Part model, mm, in its own coordinate system. Face numbers are marked on the shaded views. A direction names the side the tool comes from. Round coordinates to 2 decimals unless told otherwise and drop trailing zeros. Loops run counter-clockwise (first coordinate to the right, second up) from the corner with the lowest first, then second, coordinate; pieces in that order, holes last. Notation, with made-up numbers: (30, -32.75) -> (69, -32.75) arc R9 ccw to (69, -22.75) -> close; hole circle Ø2 at (68.25, 61.25). An arc over 180 degrees is marked (long way). Answer as a JSON object with one key per item and string values. Group by question number.
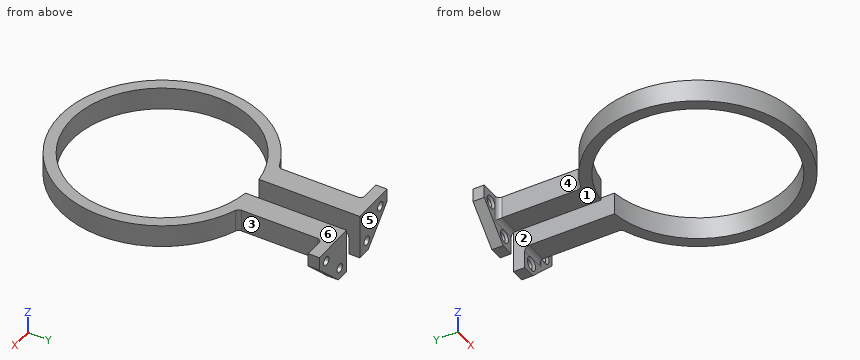
from build123d import *
from OCP.BRepFilletAPI import BRepFilletAPI_MakeChamfer

# Parameters (mm, degrees)
BOSS_EXTRUDE1_DEPTH = 12.7
SKETCH2_W           = 25.4
SKETCH2_H           = 25.4
SKETCH2_R           = 2.54
BOSS_EXTRUDE2_DEPTH = 6.35
CHAMFER2_SIZE       = 1.27
CHAMFER2_SIZE2      = 1.103994157
CHAMFER3_SIZE       = 17.78
FILLET3_R           = 2.54


with BuildPart() as part:
    # Sketch1 → Boss-Extrude1 (new body)
    with BuildSketch(Plane.XY):
        with BuildLine():
            Line((-6.35, 51.041519619), (-6.35, 101.841519619))
            Line((-6.35, 101.841519619), (-19.05, 101.841519619))
            Line((-19.05, 101.841519619), (-19.05, 54.554593986))
            ThreePointArc((-19.05, 54.554593986), (0, -57.785), (19.05, 54.554593986))
            Line((19.05, 54.554593986), (19.05, 101.841519619))
            Line((19.05, 101.841519619), (6.35, 101.841519619))
            Line((6.35, 101.841519619), (6.35, 51.041519619))
            ThreePointArc((6.35, 51.041519619), (0, -51.435), (-6.35, 51.041519619))
        make_face()
    extrude(amount=BOSS_EXTRUDE1_DEPTH)

    # Sketch2 → Boss-Extrude2 (add)
    with BuildSketch(Plane(origin=(0, 101.841519619, 0), x_dir=(1, 0, 0), z_dir=(0, 1, 0))):
        with Locations((-19.05, 0)):
            Rectangle(SKETCH2_W, SKETCH2_H)
        with Locations(Location((-25.4, -6.35, 0), (0, 0, 270))):
            Circle(SKETCH2_R, mode=Mode.SUBTRACT)
        with Locations(Location((-12.7, 6.35, 0), (0, 0, 270))):
            Circle(SKETCH2_R, mode=Mode.SUBTRACT)
    boss_extrude2 = extrude(amount=BOSS_EXTRUDE2_DEPTH)

    # Mirror5: Boss-Extrude2 across plane
    add(boss_extrude2.mirror(Plane(origin=(0, 0, 0), x_dir=(0, 0, 1), z_dir=(1, 0, 0))))

    # Chamfer2: one chamfer whose edges measure the first distance from different faces: ONE call of the kernel's chamfer builder (chamfer() names one face for all edges)
    chamfer2_edges_1 = [part.edges().sort_by_distance(p)[0] for p in [
        (-12.7, 101.841519619, -8.89),
    ]]
    chamfer2_side_1 = [part.faces().sort_by_distance(p)[0] for p in [
        (-12.7, 105.016519619, -8.89),
    ]]
    chamfer2_edges_2 = [part.edges().sort_by_distance(p)[0] for p in [
        (-25.4, 101.841519619, 3.81),
    ]]
    chamfer2_side_2 = [part.faces().sort_by_distance(p)[0] for p in [
        (-25.4, 105.016519619, 3.81),
    ]]
    chamfer2_edges_3 = [part.edges().sort_by_distance(p)[0] for p in [
        (12.7, 101.841519619, -8.89),
        (25.4, 101.841519619, 3.81),
    ]]
    chamfer2_side_3 = [part.faces().sort_by_distance(p)[0] for p in [
        (21.360206035, 101.841519619, -2.310206035),
    ]]
    chamfer2 = BRepFilletAPI_MakeChamfer(part.part.solid().wrapped)
    for e in chamfer2_edges_1:
        chamfer2.Add(CHAMFER2_SIZE, CHAMFER2_SIZE2, e.wrapped, chamfer2_side_1[0].wrapped)  # the first distance lies on this face
    for e in chamfer2_edges_2:
        chamfer2.Add(CHAMFER2_SIZE, CHAMFER2_SIZE2, e.wrapped, chamfer2_side_2[0].wrapped)  # the first distance lies on this face
    for e in chamfer2_edges_3:
        chamfer2.Add(CHAMFER2_SIZE, CHAMFER2_SIZE2, e.wrapped, chamfer2_side_3[0].wrapped)  # the first distance lies on this face
    add(Compound.cast(chamfer2.Shape()), mode=Mode.REPLACE)

    # Chamfer3
    chamfer3_edges = [part.edges().sort_by_distance(p)[0] for p in [
        (-31.75, 105.016519619, -12.7),
        (31.75, 105.016519619, -12.7),
    ]]
    chamfer(chamfer3_edges, length=CHAMFER3_SIZE)

    # Fillet3
    fillet3_edges = [part.edges().sort_by_distance(p)[0] for p in [
        (12.7, 101.841519619, 0),
        (-19.05, 54.554593986, 6.35),
        (-19.05, 101.841519619, 6.35),
        (19.05, 101.841519619, 6.35),
        (19.05, 54.554593986, 6.35),
        (-12.7, 101.841519619, 0),
    ]]
    fillet(fillet3_edges, radius=FILLET3_R - 0.0001)  # a hair under: the kernel refuses the full size


solid = part.part
Item 1: Drop flat-ended pins along their axis: pin 1 Ø1.9 at (y, z) = (106, 9.5) entering from -X; pin 2 Ø12 at (x, z) = (6, -4) entering from -Y; pin 3 Ø4 at (y, z) = (-10.5, 3.5) entering from -X; pin 4 Ø6 at (x, z) = (-25.4, 6.35) entering from +Y. Give the stop position or say it passes through.
Item 2: Band-saw the part on C-C, the plane x = -25.4. List the corners of the cut face in (y, z), plus the area to 3 significant figures.
Item 3: Which spindle directions (+Z, -Z, +X, -X, +Y, -Y) get a long thin tool onto all of the face, cutting with end or side? Do the marked faces 1, 2 and 3. Say none if no direction does.
Item 4: Band-saw the part on B-B, the plane y = 74. List the corners of the cut face in (x, z), plus the area to 3 significant figures.
Item 5: Drill centre lines: line 1 (X direction, y = 104.55, z = 6.35); line 2 (X direction, y = 60.5, z = 3); line 3 (Z direction, x = 12.7, y = 105.8). Where is each one in solid material? Low to high.
Item 6: Band-saw the part on A-A, the plane z = -6.35. List the corners of the cut face in (x, y), plus the area to 3 significant figures.
Item 7: Two-plate mould, pull along Y, no slides. Class the marked faces 4, 5 and 6: pulls with the +Y half, pulls with the -Y half, needs draft (parallel to the pull), parting line crosses it, or undercut.
Item 8: Band-saw the part on D-D, the plane y = 0. List the corners of the cut face in (x, z) (3 decimals).
Entries:
{
 "1": {"pin 1": "x = -31.75", "pin 2": "y = -57.76", "pin 3": "x = -57.16", "pin 4": "y = 108.19"},
 "2": {"outline": "(-51.9, 0) -> (-44.73, 0) -> (-44.73, 12.7) -> (-51.9, 12.7) -> close; (44.73, 0) -> (51.9, 0) -> (51.9, 12.7) -> (44.73, 12.7) -> close; (101.84, -1.27) -> (108.19, -1.27) -> (108.19, 3.81) -> (103.11, 3.81) -> (101.84, 2.71) -> close; (101.84, 9.99) -> (103.11, 8.89) -> (108.19, 8.89) -> (108.19, 12.7) -> (101.84, 12.7) -> close", "area": "237 mm²"},
 "3": {"face 1": "-Z, +X, -X, -Y", "face 2": "+Z, -Z, +Y", "face 3": "+Z, -Z, +X"},
 "4": {"outline": "(-19.05, 0) -> (-6.35, 0) -> (-6.35, 12.7) -> (-19.05, 12.7) -> close; (6.35, 0) -> (19.05, 0) -> (19.05, 12.7) -> (6.35, 12.7) -> close", "area": "323 mm²"},
 "5": {"line 1": "-31.75 to -27.94, -22.86 to -6.35, 6.35 to 22.86, 27.94 to 31.75", "line 2": "-19.05 to -6.35, 6.35 to 19.05", "line 3": "-12.7 to -8.89, -3.81 to 12.7"},
 "6": {"outline": "(-20.32, 101.84) -> (-16.34, 101.84) -> (-15.24, 103.11) -> (-15.24, 108.19) -> (-20.32, 108.19) -> close; (-10.16, 103.11) -> (-9.06, 101.84) -> (-6.35, 101.84) -> (-6.35, 108.19) -> (-10.16, 108.19) -> close; (6.35, 101.84) -> (8.89, 101.84) -> (10.16, 102.95) -> (10.16, 108.19) -> (6.35, 108.19) -> close; (15.24, 102.95) -> (16.51, 101.84) -> (20.32, 101.84) -> (20.32, 108.19) -> (15.24, 108.19) -> close", "area": "110 mm²"},
 "7": {"face 4": "undercut", "face 5": "pulls with the +Y half", "face 6": "needs draft"},
 "8": {"outline": "(-57.785, 0) -> (-51.435, 0) -> (-51.435, 12.7) -> (-57.785, 12.7) -> close; (51.435, 0) -> (57.785, 0) -> (57.785, 12.7) -> (51.435, 12.7) -> close"}
}
